Model file for the job. Use its own axes, mm. A direction names the side the tool comes from. Give positions to 0.01 mm unless a question says otherwise; leave off trailing zeros. Write each loop counter-clockwise with the first axis right and the second up, starting at its lowest first coordinate (ties: lowest second). Pieces come first, ordered by that corner, then holes. Notation, with made-up numbers: (39.25, 20) - (44.25, 20) arc R23 cw to (44.25, 44) - close; hole circle Ø11 at (12.5, 69). An arc over 180 degrees is marked (long way). Use a Markdown table: item, result. Add a question column.
```python
from build123d import *

# Parameters (mm, degrees)
SKETCH1_W                = 40
SKETCH1_H                = 46
BOSS_EXTRUDE1_DEPTH      = 46
BOSS_EXTRUDE2_DEPTH      = 10
BOSS_EXTRUDE2_DEPTH_BACK = 56
SKETCH2_R                = 15
SKETCH2_R_2              = 7.5
BOSS_EXTRUDE3_DEPTH      = 22
BOSS_EXTRUDE3_DEPTH_BACK = 62
SKETCH3_R                = 15
SKETCH3_R_2              = 9
SKETCH4_R                = 9
CUT_EXTRUDE1_DEPTH       = 130
SKETCH5_R                = 7.5
CUT_EXTRUDE2_DEPTH       = 130
SKETCH6_W                = 24
SKETCH6_H                = 30
CUT_EXTRUDE3_DEPTH       = 130


with BuildPart() as part:
    # Sketch1 → Boss-Extrude1 (new body)
    with BuildSketch(Plane.XY):
        with Locations((20, 23)):
            Rectangle(SKETCH1_W, SKETCH1_H)
    extrude(amount=BOSS_EXTRUDE1_DEPTH)

    # Sketch2 → Boss-Extrude2 (add, two sides: drawn at the far end of the back side and taken through both)
    with BuildSketch(Plane(origin=(0, 46, 0), x_dir=(1, 0, 0), z_dir=(0, 1, 0)).offset(-BOSS_EXTRUDE2_DEPTH_BACK)):
        with Locations(Location((20, -23, 0), (0, 0, 270))):
            Circle(SKETCH2_R)
        with Locations(Location((20, -23, 0), (0, 0, 270))):
            Circle(SKETCH2_R_2, mode=Mode.SUBTRACT)
    extrude(amount=BOSS_EXTRUDE2_DEPTH + BOSS_EXTRUDE2_DEPTH_BACK)

    # Sketch3 → Boss-Extrude3 (add, two sides: drawn at the far end of the back side and taken through both)
    with BuildSketch(Plane(origin=(40, 0, 0), x_dir=(0, 0, -1), z_dir=(1, 0, 0)).offset(-BOSS_EXTRUDE3_DEPTH_BACK)):
        with Locations((-23, 23)):
            Circle(SKETCH3_R)
        with Locations((-23, 23)):
            Circle(SKETCH3_R_2, mode=Mode.SUBTRACT)
    extrude(amount=BOSS_EXTRUDE3_DEPTH + BOSS_EXTRUDE3_DEPTH_BACK)

    # Sketch4 → Cut-Extrude1 (cut)
    with BuildSketch(Plane(origin=(40, 0, 0), x_dir=(0, 0, -1), z_dir=(1, 0, 0))):
        with Locations((-23, 23)):
            Circle(SKETCH4_R)
    extrude(amount=-CUT_EXTRUDE1_DEPTH, mode=Mode.SUBTRACT)

    # Sketch5 → Cut-Extrude2 (cut)
    with BuildSketch(Plane(origin=(0, 46, 0), x_dir=(1, 0, 0), z_dir=(0, 1, 0))):
        with Locations(Location((20, -23, 0), (0, 0, 270))):
            Circle(SKETCH5_R)
    extrude(amount=-CUT_EXTRUDE2_DEPTH, mode=Mode.SUBTRACT)

    # Sketch6 → Cut-Extrude3 (cut)
    with BuildSketch(Plane.XY.offset(46)):
        with Locations((20, 23)):
            Rectangle(SKETCH6_W, SKETCH6_H)
    extrude(amount=-CUT_EXTRUDE3_DEPTH, mode=Mode.SUBTRACT)


solid = part.part
```
(1) Two-plate mould, pull along Z, no slides. Class faces 4 (the cylindrical face through (5.357, 50.93, 19.748)), 5 (the flat face through (40, 23, 7)), 6 (the cylindrical face through (25.1, 47.1, 17.5)), 7 (the cylindrical face through (-7.21, 25.703, 14.416)): +Z half, -Z half, draft (parallel to the pull), parting line (faces both ways), or undercut.
(2) Probe probe 1 along X at (y, z) = (28.5, 7); probe 2 along X at (y, z) = (-2, 23); probe 3 along Z at (x, y) = (41.5, 23). List the from-to ranges inside material, lowest first. Write a range as [from, to].
(3) Band-saw the part on C-C (y = 31). Write the cut outline in (x, z).
(4) Band-saw the part on D-D (x = 6). Write the cut outline in (y, z), then the cut area to 3 significant figures.
(5) Band-saw the part on B-B (z = 39.5). Write the cut outline in (x, y), then the cut area to 3 significant figures.
(6) Which spindle directions (+Z, -Z, +X, -X, +Y, -Y) get a long thin tool onto all of the face, cutting with end or side? Do faces 1 (the cylindrical face through (50.846, 8.357, 26.252)), 2 (the flat face through (14, 8, 28)), 3 (the flat face through (20, 46, 7)). Say none if no direction does.
(7) Band-saw the part on A-A (x = 20). Write the cut outline in (y, z).
(8) Flat gauge pins, fed straight in: pin 1 (4 mm diameter, centred on x = 34.5, z = 9, fed in from +Y); pin 2 (2 mm diameter, centred on y = -3.5, z = 14.5, fed in from +X); pin 3 (6 mm diameter, centred on x = -11, y = 12, fed in from +Z). Where does each tip first touch, or does it go through?
Model answer:
| question | item | result |
|---|---|---|
| 1 | face 4 | parting line |
| 1 | face 5 | draft |
| 1 | face 6 | undercut |
| 1 | face 7 | undercut |
| 2 | probe 1 | x = [0, 8], [32, 40] |
| 2 | probe 2 | x = [5, 12.5], [27.5, 35] |
| 2 | probe 3 | z = [8, 14], [32, 38] |
| 3 | outline | (-22, 10.31) - (0, 10.31) - (0, 0) - (8, 0) - (8, 18.88) - (-22, 18.88) - close; (-22, 27.12) - (8, 27.12) - (8, 46) - (0, 46) - (0, 35.69) - (-22, 35.69) - close; (32, 0) - (40, 0) - (40, 10.31) - (62, 10.31) - (62, 18.88) - (32, 18.88) - close; (32, 27.12) - (62, 27.12) - (62, 35.69) - (40, 35.69) - (40, 46) - (32, 46) - close |
| 4 | outline | (-10, 17.61) - (0, 17.61) - (0, 0) - (46, 0) - (46, 17.61) - (56, 17.61) - (56, 28.39) - (46, 28.39) - (46, 46) - (0, 46) - (0, 28.39) - (-10, 28.39) - close; hole circle Ø18 at (23, 23) |
| 4 | area | 2,080 mm^2 |
| 5 | outline | (0, 0) - (40, 0) - (40, 46) - (0, 46) - close; hole (8, 8) - (32, 8) - (32, 38) - (8, 38) - close |
| 5 | area | 1,120 mm^2 |
| 6 | face 1 | +X |
| 6 | face 2 | +Z, -Z |
| 6 | face 3 | +Y |
| 7 | outline | (-10, 8) - (0, 8) - (0, 0) - (8, 0) - (8, 15.5) - (-10, 15.5) - close; (-10, 30.5) - (8, 30.5) - (8, 46) - (0, 46) - (0, 38) - (-10, 38) - close; (38, 0) - (46, 0) - (46, 8) - (56, 8) - (56, 15.5) - (38, 15.5) - close; (38, 30.5) - (56, 30.5) - (56, 38) - (46, 38) - (46, 46) - (38, 46) - close |
| 8 | pin 1 | stops at y = 46 |
| 8 | pin 2 | stops at x = 32.99 |
| 8 | pin 3 | stops at z = 35.69 |
